from build123d import *

# Parameters (mm, degrees)
SKETCH1_W           = 42
SKETCH1_H           = 42
NEMA_17_DEPTH       = 9
CHAMFER1_SIZE       = 5.5
SKETCH2_R           = 3
M6_BOLT_HOLES_DEPTH = 8
SKETCH3_W           = 16
SKETCH3_H           = 3
BOSS_EXTRUDE1_DEPTH = 4
SKETCH5_W           = 16
SKETCH5_H           = 5
BOSS_EXTRUDE2_DEPTH = 6
SKETCH6_W           = 14
SKETCH6_H           = 3
CUT_EXTRUDE1_DEPTH  = 5
SKETCH7_W           = 4.019368502
SKETCH7_H           = 10
CUT_EXTRUDE2_DEPTH  = 1
SKETCH8_W           = 1.150216319
SKETCH8_H           = 0.828591851
SKETCH8_W_2         = 1.150216318
BOSS_EXTRUDE3_DEPTH = 5
CHAMFER2_SIZE       = 0.3


with BuildPart() as part:
    # Sketch1 → Nema 17 (new body)
    with BuildSketch(Plane(origin=(0, 0, 0), x_dir=(1, 0, 0), z_dir=(0, 1, 0))):
        Rectangle(SKETCH1_W, SKETCH1_H)
    extrude(amount=NEMA_17_DEPTH)

    # Chamfer1
    chamfer1_edges = [part.edges().sort_by_distance(p)[0] for p in [
        (21, 4.5, 21),
        (-21, 4.5, 21),
        (-21, 4.5, -21),
        (21, 4.5, -21),
    ]]
    chamfer(chamfer1_edges, length=CHAMFER1_SIZE)

    # Sketch2 → M6 Bolt Holes (cut)
    with BuildSketch(Plane.XZ):
        with Locations(Location((-15.5, -15.5, 0), (0, 0, 270))):
            Circle(SKETCH2_R)
        with Locations(Location((15.5, -15.5, 0), (0, 0, 90))):
            Circle(SKETCH2_R)
        with Locations(Location((-15.5, 15.5, 0), (0, 0, 90))):
            Circle(SKETCH2_R)
        with Locations(Location((15.5, 15.5, 0), (0, 0, 270))):
            Circle(SKETCH2_R)
    extrude(amount=-M6_BOLT_HOLES_DEPTH, mode=Mode.SUBTRACT)

    # Sketch3 → Boss-Extrude1 (add)
    with BuildSketch(Plane.ZY.offset(21)):
        with Locations((0, 1.5)):
            Rectangle(SKETCH3_W, SKETCH3_H)
    extrude(amount=BOSS_EXTRUDE1_DEPTH)

    # Sketch5 → Boss-Extrude2 (add)
    with BuildSketch(Plane.ZY.offset(21)):
        with Locations((0, 7.5)):
            Rectangle(SKETCH5_W, SKETCH5_H)
    extrude(amount=BOSS_EXTRUDE2_DEPTH)

    # Sketch6 → Cut-Extrude1 (cut)
    with BuildSketch(Plane.ZY.offset(27)):
        with Locations((0, 7.5)):
            Rectangle(SKETCH6_W, SKETCH6_H)
    extrude(amount=-CUT_EXTRUDE1_DEPTH, mode=Mode.SUBTRACT)

    # Sketch7 → Cut-Extrude2 (cut)
    with BuildSketch(Plane(origin=(0, 10, 0), x_dir=(1, 0, 0), z_dir=(0, 1, 0))):
        with Locations((-24.990315749, 0)):
            Rectangle(SKETCH7_W, SKETCH7_H)
    extrude(amount=-CUT_EXTRUDE2_DEPTH, mode=Mode.SUBTRACT)

    # Sketch8 → Boss-Extrude3 (add)
    with BuildSketch(Plane.ZY.offset(22)):
        with Locations((5.539336093, 7.499295926)):
            Rectangle(SKETCH8_W, SKETCH8_H)
        with Locations((3.346490506, 7.499295926)):
            Rectangle(SKETCH8_W_2, SKETCH8_H)
        with Locations((1.15364492, 7.499295926)):
            Rectangle(SKETCH8_W, SKETCH8_H)
        with Locations((-1.039200668, 7.499295926)):
            Rectangle(SKETCH8_W, SKETCH8_H)
        with Locations((-3.232046254, 7.499295926)):
            Rectangle(SKETCH8_W_2, SKETCH8_H)
        with Locations((-5.42489184, 7.499295926)):
            Rectangle(SKETCH8_W, SKETCH8_H)
    extrude(amount=BOSS_EXTRUDE3_DEPTH)

    # Chamfer2
    chamfer2_edges = [part.edges().sort_by_distance(p)[0] for p in [
        (-27, 7.499295925, 4.964227933),
        (-27, 7.085, 5.539336093),
        (-27, 7.499295925, 6.114444252),
        (-27, 7.913591851, 5.539336093),
        (-27, 7.913591851, 3.346490506),
        (-27, 7.499295925, 2.771382347),
        (-27, 7.085, 3.346490506),
        (-27, 7.499295925, 3.921598665),
        (-27, 7.913591851, 1.153644919),
        (-27, 7.499295925, 0.57853676),
        (-27, 7.085, 1.153644919),
        (-27, 7.499295925, 1.728753079),
        (-27, 7.913591851, -1.039200667),
        (-27, 7.499295925, -1.614308827),
        (-27, 7.085, -1.039200667),
        (-27, 7.499295925, -0.464092508),
        (-27, 7.913591851, -3.232046254),
        (-27, 7.499295925, -3.807154413),
        (-27, 7.085, -3.232046254),
        (-27, 7.499295925, -2.656938095),
        (-27, 7.913591851, -5.424891841),
        (-27, 7.499295925, -6),
        (-27, 7.085, -5.424891841),
        (-27, 7.499295925, -4.849783681),
    ]]
    chamfer(chamfer2_edges, length=CHAMFER2_SIZE)


solid = part.part
Design review of the part built by this model. Coordinates are the model's own, in mm. A direction names the side the tool comes from. Round coordinates to 2 decimals unless told otherwise and drop trailing zeros. Loops run counter-clockwise (first coordinate to the right, second up) from the corner with the lowest first, then second, coordinate; pieces in that order, holes last. Notation, with made-up numbers: (19, 89) - (64, 89) arc R15 ccw to (64, 110) - close; hole circle Ø4 at (74.25, -16). An arc over 180 degrees is marked (long way). One line per item, written item: value. Start each with the question number.
1) Insertion check: pin 1 Ø2.5 at (x, y) = (-24, 7.5) entering from +Z; pin 2 Ø2.5 at (x, y) = (-22.5, 2) entering from -Z; pin 3 Ø7 at (x, z) = (-15.5, -15.5) entering from +Y. Each pin has a flat end and moves straight along its axis. Give the tip position at first contact, or say it passes through.
2) To check wall thickness, follow L1, parallel to X at y = 2.75, z = -15.5; L2, parallel to Z at x = -17, y = 4.25; L3, parallel to Z at x = -16, y = 5.5. State the ranges of each line that lie inside material, in increasing order. Write a range as from..to.
3) Consider section B-B on z = -14.5. Give the boundary of the cut face in (x, y).
4) Consider section C-C on x = 11.5. Give the boundary of the cut face in (y, z).
5) Consider section A-A on y = 3.75. Give the boundary of the cut face in (x, z).
6) For faces 1 (the flat face through (-25, 9.5, 5)), 2 (the flat face through (-23, 1, 8)), 3 (the flat face through (-24, 5, 0)), 4 (the flat face through (-22.3, 9, -0.1)), list the 3-axis set-ups (+Z, -Z, +X, -X, +Y, -Y) from which the entire face can be reached by the end or side of a thin tool; tool diameter is ignored.
7) Consider section D-D on x = 17.5. Give the boundary of the cut face in (y, z), then the cut area to 3 significant figures.
8) Draft analysis for pull direction X (two halves, no side actions). For faces 5 (the flat face through (15, 8, -16)), 6 (the flat face through (21, 4, 0)), 7 (the flat face through (0, 4, 21)), state which applies: +X half, -X half, draft (parallel to the pull), parting line (faces both ways), or undercut.
Reported:
1. pin 1: stops at z = 8
1. pin 2: stops at z = -8
1. pin 3: stops at y = 9
2. L1: x = -21..-18.5, -12.5..12.5, 18.5..21
2. L2: z = -19.5..-18.1, -12.9..12.9, 18.1..19.5
2. L3: z = -20.5..-18.46, -12.54..12.54, 18.46..20.5
3. outline: (-21, 0) - (-18.33, 0) - (-18.33, 8) - (-12.67, 8) - (-12.67, 0) - (12.67, 0) - (12.67, 8) - (18.33, 8) - (18.33, 0) - (21, 0) - (21, 9) - (-21, 9) - close
4. outline: (0, -21) - (9, -21) - (9, 21) - (0, 21) - close
5. outline: (-21, -15.5) - (-15.5, -21) - (15.5, -21) - (21, -15.5) - (21, 15.5) - (15.5, 21) - (-15.5, 21) - (-21, 15.5) - close; hole circle Ø6 at (-15.5, -15.5); hole circle Ø6 at (-15.5, 15.5); hole circle Ø6 at (15.5, -15.5); hole circle Ø6 at (15.5, 15.5)
6. face 1: -X, +Y
6. face 2: +Z, -X, +Y, -Y
6. face 3: +Z, -Z, -X
6. face 4: -X
7. outline: (0, -19) - (9, -19) - (9, 19) - (0, 19) - (0, 17.74) - (8, 17.74) - (8, 13.26) - (0, 13.26) - (0, -13.26) - (8, -13.26) - (8, -17.74) - (0, -17.74) - close
7. area: 270 mm^2
8. face 5: undercut
8. face 6: +X half
8. face 7: draft
